Autodesk Inventor part; units mm, degrees
ref_plane "YZ Plane" through (0, 0, 0) normal (1, 0, 0) x (0, 1, 0)
ref_plane "XZ Plane" through (0, 0, 0) normal (0, 1, 0) x (-1, 0, 0)
ref_plane "XY Plane" through (0, 0, 0) normal (0, 0, 1) x (1, 0, 0)
sketch "Sketch1" plane through (0, 0, 0) normal (0, 1, 0) x (-1, 0, 0)
  line L0 (0, 0) -> (127, 0)
  line L1 (127, 0) -> (127, -177.8)
  line L2 (127, -177.8) -> (0, -177.8)
  line L3 (0, -177.8) -> (0, 0)
  dimension "d0" = 127
  dimension "d1" = 177.8
extrude "Extrusion1" add sketch "Sketch1" along normal blind 1.5875
sketch "Sketch2" plane through (0, 1.5875, 0) normal (0, 1, 0) x (1, 0, 0)
  line L0 (-127, 177.8) -> (-127, 0)
  line L1 (0, 177.8) -> (-127, 177.8)
  line L2 (0, 0) -> (0, 177.8)
  line L3 (-127, 0) -> (0, 0)
  point P0 (-121.92, 172.72)
  point P1 (-5.08, 172.72)
  point P2 (-5.08, 5.08)
  point P3 (-121.92, 5.08)
  dimension "d4" = 5.08
  dimension "d5" = 5.08
  dimension "d6" = 5.08
  dimension "d7" = 5.08
  dimension "d8" = 5.08
  dimension "d9" = 5.08
  dimension "d10" = 5.08
  dimension "d11" = 5.08
hole "Hole1" at (-121.92, 1.5875, -172.72) at (-5.08, 1.5875, -172.72) at (-5.08, 1.5875, -5.08) at (-121.92, 1.5875, -5.08) direction (0, -1, 0) diameter 3.5 end through all
sketch "Sketch3" plane through (0, 1.5875, 0) normal (0, 1, 0) x (1, 0, 0)
  circle A0 centre (-5.08, 5.08) radius 1.75
  circle A1 centre (-121.92, 172.72) radius 1.75
  circle A2 centre (-5.08, 172.72) radius 1.75
  circle A3 centre (-121.92, 5.08) radius 1.75
  line L0 (-127, 0) -> (0, 0)
  line L1 (0, 0) -> (0, 177.8)
  line L2 (0, 177.8) -> (-127, 177.8)
  line L3 (-127, 177.8) -> (-127, 0)
  line L4 (-127, 0) -> (0, 0)
  line L5 (0, 177.8) -> (-127, 177.8)
  line L6 (-28.9, 0) -> (-25.4, 0)
  line L7 (-25.4, 0) -> (-25.4, 177.8)
  line L8 (-25.4, 177.8) -> (-28.9, 177.8)
  line L9 (-28.9, 177.8) -> (-28.9, 0)
  dimension "d19" = 3.5
  dimension "d23" = 25.4
extrude "Extrusion2" add sketch "Sketch3" along normal blind 2.54 contours L9 L2 L7 L0
properties part number "MockPCB"
Could you check a few things on this model? Use its own coordinates, in mm. A direction names the side the tool comes from. Give positions to 0.01 mm unless a question says otherwise; leave off trailing zeros. Order: outer loops, then holes, each group sorted by start corner. A loop starts at its lowest first (then second) coordinate and runs counter-clockwise, first axis right, second up. Notation, with made-up numbers: M 71.25,34 L 122.25,34 A18 cw 122.25,49 Z; hole C 24.5,87.25 d11. An arc over 180 degrees is marked long. One line per question, with ' | ' between items.
1. If I drill on line 1 (Z direction, x = -5.08, y = 1.1); line 2 (X direction, y = 1, z = -5.08); line 3 (X direction, y = 2.6, z = -59.5), over which ranges is the centre line in solid material (lowest first)?
Results:
line 1: -177.8 to -174.47, -170.97 to -6.83, -3.33 to 0 | line 2: -127 to -123.67, -120.17 to -6.83, -3.33 to 0 | line 3: -28.9 to -25.4
2. For faces 5 (the face through (-64, 1, -177.8)), 6 (the face through (-77, 1.588, -88)), 7 (the face through (-13, 1.588, -88)), which set-ups out of +Z, -Z, +X, -X, +Y, -Y let a thin tool reach every point of the face, with its end or its side?
Results:
face 5: -Z, +X, -X, +Y, -Y | face 6: +Z, -Z, -X, +Y | face 7: +Z, -Z, +X, +Y
3. I want a section at A-A (z = -172.72). List the corners of the cut face in (x, y) for me.
Results:
outline: M -127,0 L -123.67,0 L -123.67,1.59 L -127,1.59 Z; M -120.17,0 L -6.83,0 L -6.83,1.59 L -25.4,1.59 L -25.4,4.13 L -28.9,4.13 L -28.9,1.59 L -120.17,1.59 Z; M -3.33,0 L 0,0 L 0,1.59 L -3.33,1.59 Z
4. We'd pull the mould along Z, two halves only. Please class faces 1 (the face through (-123.655, 0.783, -5.308)), 2 (the face through (-63, 0, -88)), 3 (the face through (-63, 1, 0)), 4 (the face through (-5.606, 0.783, -171.051)): +Z half, -Z half, draft (parallel to the pull), parting line (faces both ways), or undercut.
Results:
face 1: undercut | face 2: draft | face 3: +Z half | face 4: undercut
5. I want a section at D-D (x = -105). List the corners of the cut face in (y, z) for me, and give its area (3 significant figures).
Results:
outline: M 0,-177.8 L 1.59,-177.8 L 1.59,0 L 0,0 Z | area: 282 mm²
6. I want a section at C-C (z = -32). List the corners of the cut face in (x, y) for me, and give its area (3 significant figures).
Results:
outline: M -127,0 L 0,0 L 0,1.59 L -25.4,1.59 L -25.4,4.13 L -28.9,4.13 L -28.9,1.59 L -127,1.59 Z | area: 211 mm²
7. I'm going to push flat-ended pins straight in: pin 1 (1 mm diameter, centred on x = -100.5, z = -104, fed in from +Y); pin 2 (1 mm diameter, centred on x = -109.5, z = -28, fed in from -Y); pin 3 (1.3 mm diameter, centred on y = 2.5, z = -60.5, fed in from +X). Where does each tip first touch, or does it pass through?
Results:
pin 1: y = 1.59 | pin 2: y = 0 | pin 3: x = -25.4
8. I want a section at B-B (x = -121.92). List the corners of the cut face in (y, z) for me.
Results:
outline: M 0,-177.8 L 1.59,-177.8 L 1.59,-174.47 L 0,-174.47 Z; M 0,-170.97 L 1.59,-170.97 L 1.59,-6.83 L 0,-6.83 Z; M 0,-3.33 L 1.59,-3.33 L 1.59,0 L 0,0 Z
